```python
from build123d import *

# Parameters (mm, degrees)
F3_R     = 19.05
F4_DEPTH = 19.05
F6_DEPTH = 6.35
F7_R     = 2.54
F8_DEPTH = 8.891


with BuildPart() as f1:
    # F0 (on Front) → F1 (revolve)
    with BuildSketch(Plane.XZ):
        with BuildLine():
            Line((0, 57.15), (0, 0))
            Line((0, 0), (8.89, 0))
            Line((8.89, 0), (8.89, 57.15))
            Line((8.89, 57.15), (7.62, 57.15))
            ThreePointArc((7.62, 57.15), (6.35, 55.88), (5.08, 57.15))
            Line((5.08, 57.15), (3.81, 57.15))
            ThreePointArc((3.81, 57.15), (2.54, 55.88), (1.27, 57.15))
            Line((1.27, 57.15), (0, 57.15))
        make_face()
    revolve(axis=Axis((4.445, 0, 0), (1, 0, 0)))

    # F3 (on face) → F4 (cut)
    with BuildSketch(Plane.YZ.offset(8.89)):
        with Locations((-31.75, 0)):
            Circle(F3_R)
        with Locations((0, 31.75)):
            Circle(F3_R)
        with Locations((31.75, 0)):
            Circle(F3_R)
        with Locations((0, -31.75)):
            Circle(F3_R)
    extrude(amount=-F4_DEPTH, mode=Mode.SUBTRACT)

    # F5 (on Right) → F6 (cut)
    with BuildSketch(Plane.YZ):
        Polygon((-6.223, 3.592851), (-6.223, -3.592851), (0, -7.185701), (6.223, -3.592851), (6.223, 3.592851), (0, 7.185701), align=None)
    extrude(amount=F6_DEPTH, mode=Mode.SUBTRACT)

    # F7 (on face) → F8 (cut, through all)
    with BuildSketch(Plane.YZ.offset(8.89)):
        Circle(F7_R)
    extrude(amount=-F8_DEPTH, mode=Mode.SUBTRACT)


solid = f1.part
```
Could you check a few things on this model? Use its own coordinates, in mm. A direction names the side the tool comes from. Round coordinates to 2 decimals unless told otherwise and drop trailing zeros. Loops run counter-clockwise (first coordinate to the right, second up) from the corner with the lowest first, then second, coordinate; pieces in that order, holes last. Notation, with made-up numbers: (-0.75, 57) -> (17.25, 57) arc R22 ccw to (17.25, 88) -> close; hole circle Ø1 at (72.5, -26.5). An arc over 180 degrees is marked (long way). Put each result on its own line as item: value.
Q1. For pin 1 Ø2 at (y, z) = (-18.5, 39) entering from -X; pin 2 Ø5 at (x, z) = (2, 1.5) entering from -Y; pin 3 Ø1 at (x, z) = (5, 27.5) entering from -Y; pin 4 Ø1.9 at (x, z) = (4, -1.5) entering from +Y, each with a flat end and sliding along its axis, tell me the tip position at first contact or that it passes through.
Checks:
pin 1: x = 0
pin 2: y = -57.15
pin 3: y = -50.37
pin 4: y = 57.15
Q2. I want a section at B-B on y = -15.5. Give the number of separate pieces and of enclosed holes in the cut face, and give its area (3 significant figures).
Checks:
separate pieces: 4
enclosed holes: 0
area: 397 mm2
Q3. Thinking about a two-plate mould opening in Y: for faces 1 (the cylindrical face through (8.246, -2.513, -57.095)), 2 (the flat face through (3, 6.223, 0)), 3 (the flat face through (0, 12, -1)), which applies, pulls with the +Y half, pulls with the -Y half, needs draft (parallel to the pull), parting line crosses it, or undercut?
Checks:
face 1: parting line crosses it
face 2: undercut
face 3: needs draft
Q4. Please list where these lines run through material, in increasing order: line 1 (Z direction, x = 4.75, y = 4); line 2 (Y direction, x = 7.5, z = 3); line 3 (Y direction, x = 1.5, z = -8.5). Write a range as from..to.
Checks:
line 1: -57.01..-50.38, -13.12..-4.88, 4.88..13.12, 50.38..57.01
line 2: -56.53..-50.56, -12.94..12.94, 50.56..56.53
line 3: -55.78..-48.8, -14.7..14.7, 48.8..55.78
Q5. I want a section at A-A on z = 0. Write out the boundary of the cut face in (x, y), and give its area (3 significant figures).
Checks:
outline: (0, -57.15) -> (1.27, -57.15) arc R1.27 cw to (3.81, -57.15) -> (5.08, -57.15) arc R1.27 cw to (7.62, -57.15) -> (8.89, -57.15) -> (8.89, -50.8) -> (0, -50.8) -> close; (0, -12.7) -> (8.89, -12.7) -> (8.89, -2.54) -> (6.35, -2.54) -> (6.35, -6.22) -> (0, -6.22) -> close; (0, 6.22) -> (6.35, 6.22) -> (6.35, 2.54) -> (8.89, 2.54) -> (8.89, 12.7) -> (0, 12.7) -> close; (0, 50.8) -> (8.89, 50.8) -> (8.89, 57.15) -> (7.62, 57.15) arc R1.27 cw to (5.08, 57.15) -> (3.81, 57.15) arc R1.27 cw to (1.27, 57.15) -> (0, 57.15) -> close
area: 237 mm2
Q6. Which directions (+Z, -Z, +X, -X, +Y, -Y) give clear straight access to the entire face, cutting with the end or side of a thin tool? Please do faces 4 (the flat face through (8.89, 12, 1)), 5 (the flat face through (3.13, -3.16, -5.36)).
Checks:
face 4: +Z, -Z, +X, +Y, -Y
face 5: -X
